Here's the drawing with two shaded views (mm, measured from the low corner). I have some questions. Give positions to 0.01 mm unless a question says otherwise; leave off trailing zeros. Write each loop counter-clockwise with the first axis right and the second up, starting at its lowest first coordinate (ties: lowest second). Pieces come first, ordered by that corner, then holes.
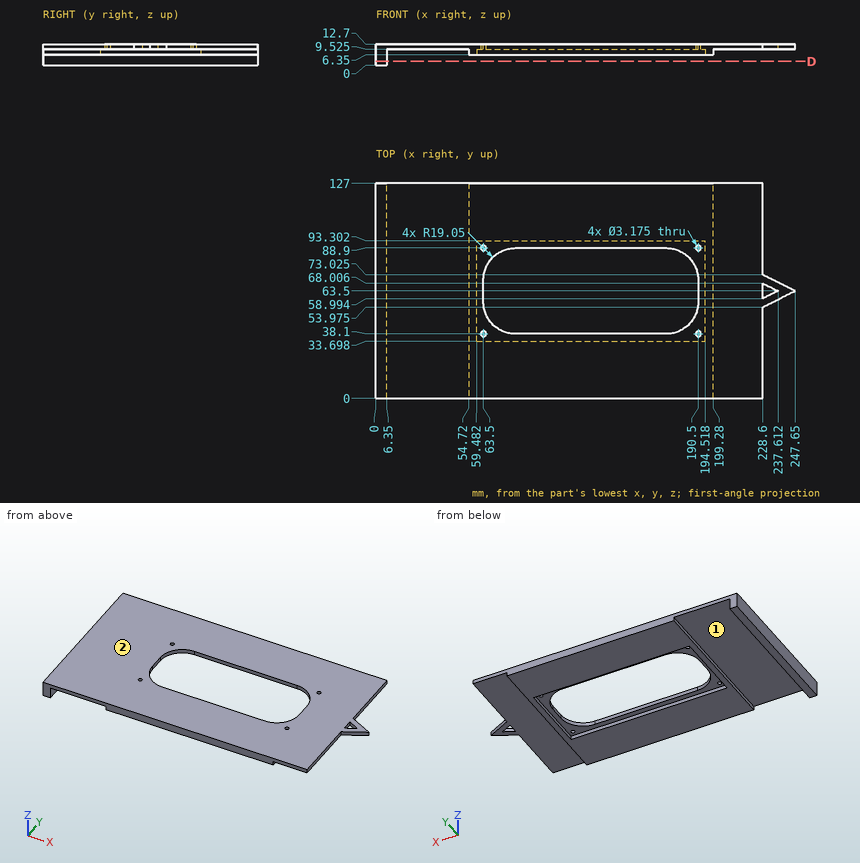
(1) Will these pins go through, and if not, where does the flat tip stop? P1, Ø2.5, axis at y = 62.5, z = 10.5, coming from the +X side; P2, Ø3, axis at x = 90.5, y = 20, coming from the -Z side; P3, Ø1.9, axis at x = 63.5, y = 38.1, coming from the -Z side; P4, Ø14.5, axis at x = 21, y = 68.5, coming from the -Z side (3 decimals).
Returned:
P1: stops at x = 247.65
P2: stops at z = 6.35
P3: passes through
P4: stops at z = 9.525
(2) If we mould it in two halves opening along X, with no side actions, what happens to the marked faces 1 and 2? For each: +X half, -X half, draft (parallel to the pull), parting line (faces both ways), or undercut.
Returned:
face 1: undercut
face 2: draft
(3) Imagine slicing it at D-D, the plane z = 2.5. Write out the boundary of the cut face in (x, y).
Returned:
outline: (0, 0) - (6.35, 0) - (6.35, 127) - (0, 127) - close
(4) If I drill on L1, parallel to X at y = 75, z = 7; L2, parallel to Y at x = 115.5, z = 11.75; L3, parallel to Z at x = 55, y = 33.5, over which ranges is the centre line in solid material (lowest first)?
Returned:
L1: x = 0 to 6.35, 54.72 to 59.48, 194.52 to 199.28
L2: y = 0 to 38.1, 88.9 to 127
L3: z = 6.35 to 12.7
